from build123d import *

# Parameters (mm, degrees)
F0_W     = 128.999456
F0_H     = 134.383812
F1_DEPTH = 0.4
F2_R     = 5


with BuildPart() as f1:
    # F0 (on Front) → F1 (new body)
    with BuildSketch(Plane.XZ):
        Rectangle(F0_W, F0_H)
        with BuildLine():
            Line((17.46, -61.855495), (0, -61.855495))
            Line((0, -61.855495), (-17.46, -61.855495))
            ThreePointArc((-17.46, -61.855495), (-19.256051, -61.111547), (-20, -59.315495))
            Line((-20, -59.315495), (-20, 0.418954))
            ThreePointArc((-20, 0.418954), (-20.743949, 2.215005), (-22.54, 2.958954))
            Line((-22.54, 2.958954), (-35.495363, 2.958954))
            ThreePointArc((-35.495363, 2.958954), (-37.751578, 4.332294), (-37.567989, 6.967226))
            Line((-37.567989, 6.967226), (-2.072625, 57.072777))
            ThreePointArc((-2.072625, 57.072777), (0, 58.144505), (2.072625, 57.072777))
            Line((2.072625, 57.072777), (37.567989, 6.967226))
            ThreePointArc((37.567989, 6.967226), (37.751578, 4.332294), (35.495363, 2.958954))
            Line((35.495363, 2.958954), (22.54, 2.958954))
            ThreePointArc((22.54, 2.958954), (20.743949, 2.215005), (20, 0.418954))
            Line((20, 0.418954), (20, -59.315495))
            ThreePointArc((20, -59.315495), (19.256051, -61.111547), (17.46, -61.855495))
        make_face(mode=Mode.SUBTRACT)
    extrude(amount=F1_DEPTH)

    # F2
    f2_edges = [f1.edges().sort_by_distance(p)[0] for p in [
        (-64.499728, -0.2, 67.191906),
        (64.499728, -0.2, 67.191906),
        (64.499728, -0.2, -67.191906),
        (-64.499728, -0.2, -67.191906),
    ]]
    fillet(f2_edges, radius=F2_R)


solid = f1.part
Can you work these out from the model? Positions are in its coordinate system, mm. Coordinates: 2 decimals unless noted, no trailing zeros. Write each loop counter-clockwise with the first axis right and the second up, starting at its lowest first coordinate (ties: lowest second). Pieces come first, ordered by that corner, then holes.
Q1. Imagine slicing it at B-B, the plane y = -0.3. List the corners of the cut face in (x, z) for me, plus the area to 3 significant figures.
Results found:
outline: (-64.5, -62.19) arc R5 ccw to (-59.5, -67.19) - (59.5, -67.19) arc R5 ccw to (64.5, -62.19) - (64.5, 62.19) arc R5 ccw to (59.5, 67.19) - (-59.5, 67.19) arc R5 ccw to (-64.5, 62.19) - close; hole (-37.57, 6.97) arc R2.54 ccw to (-35.5, 2.96) - (-22.54, 2.96) arc R2.54 cw to (-20, 0.42) - (-20, -59.32) arc R2.54 ccw to (-17.46, -61.86) - (17.46, -61.86) arc R2.54 ccw to (20, -59.32) - (20, 0.42) arc R2.54 cw to (22.54, 2.96) - (35.5, 2.96) arc R2.54 ccw to (37.57, 6.97) - (2.07, 57.07) arc R2.54 ccw to (-2.07, 57.07) - close
area: 12,400 mm2
Q2. Please list where these lines run through material, in increasing order: L1, parallel to X at y = -0.05, z = -40; L2, parallel to Z at x = 32, y = -0.25; L3, parallel to X at y = -0.25, z = 19.
Results found:
L1: x = -64.5 to -20, 20 to 64.5
L2: z = -67.19 to 2.96, 14.83 to 67.19
L3: x = -64.5 to -29.04, 29.04 to 64.5
Q3. Imagine slicing it at C-C, the plane x = 8. List the corners of the cut face in (y, z) for me, plus the area to 3 significant figures.
Results found:
outline: (-0.4, -67.19) - (0, -67.19) - (0, -61.86) - (-0.4, -61.86) - close; (-0.4, 48.71) - (0, 48.71) - (0, 67.19) - (-0.4, 67.19) - close
area: 9.53 mm2
Q4. If we mould it in two halves opening along X, with no side actions, what happens to faces 1 (the face through (19.57, -0.2, 32.37)), 2 (the face through (28, -0.4, 1)), 3 (the face through (-20.07, -0.2, 31.67)), 4 (the face through (-63.07, -0.2, -65.69))? For each: +X half, -X half, draft (parallel to the pull), parting line (faces both ways), or undercut.
Results found:
face 1: undercut
face 2: draft
face 3: undercut
face 4: -X half
Q5. Imagine slicing it at A-A, the plane z = -15.5. List the corners of the cut face in (x, y) for me, plus the area to 3 significant figures.
Results found:
outline: (-64.5, -0.4) - (-20, -0.4) - (-20, 0) - (-64.5, 0) - close; (20, -0.4) - (64.5, -0.4) - (64.5, 0) - (20, 0) - close
area: 35.6 mm2
